Autodesk Inventor part; units mm, degrees
ref_plane "YZ Plane" through (0, 0, 0) normal (1, 0, 0) x (0, 1, 0)
ref_plane "XZ Plane" through (0, 0, 0) normal (0, 1, 0) x (-1, 0, 0)
ref_plane "XY Plane" through (0, 0, 0) normal (0, 0, 1) x (1, 0, 0)
sketch "Sketch1" plane through (0, 0, 0) normal (0, 1, 0) x (-1, 0, 0)
  line L0 (0, 0) -> (45, 0)
  line L1 (45, 0) -> (45, -84)
  line L2 (45, -84) -> (0, -84)
  line L3 (0, -84) -> (0, 0)
  line L4 (0, 0) -> (45, 0)
  line L5 (0, 2) -> (0, 0)
  circle A0 centre (6, -74) radius 2
  circle A1 centre (39, -74) radius 2
  line L6 (22.5, 0) -> (22.5, -84)
  line L7 (45, -10) -> (0, -10)
  line L8 (6, -3.5) -> (10.7625, -3.5)
  line L9 (10.7625, -3.5) -> (10.7625, -5)
  line L10 (10.7625, -5) -> (6, -5)
  line L11 (6, -5) -> (6, -3.5)
  line L12 (6, -16.5) -> (10.7625, -16.5)
  line L13 (10.7625, -16.5) -> (10.7625, -15)
  line L14 (10.7625, -15) -> (6, -15)
  line L15 (6, -15) -> (6, -16.5)
  line L16 (39, -3.5) -> (34.2375, -3.5)
  line L17 (34.2375, -3.5) -> (34.2375, -5)
  line L18 (34.2375, -5) -> (39, -5)
  line L19 (39, -5) -> (39, -3.5)
  line L20 (34.2375, -16.5) -> (34.2375, -15)
  line L21 (39, -15) -> (39, -16.5)
  line L22 (39, -16.5) -> (34.2375, -16.5)
  line L23 (34.2375, -15) -> (39, -15)
  dimension "d0" = 45
  dimension "d1" = 84
  dimension "d3" = 10
  dimension "d4" = 6
  dimension "d5" = 10
  dimension "d6" = 6
  dimension "d7" = 4
  dimension "d8" = 4
  dimension "d19" = 20
  dimension "d20" = 6
  dimension "d21" = 10
  dimension "d22" = 1.5
extrude "Extrusion4" add sketch "Sketch1" along normal blind 1
properties part number "Platte1_2"
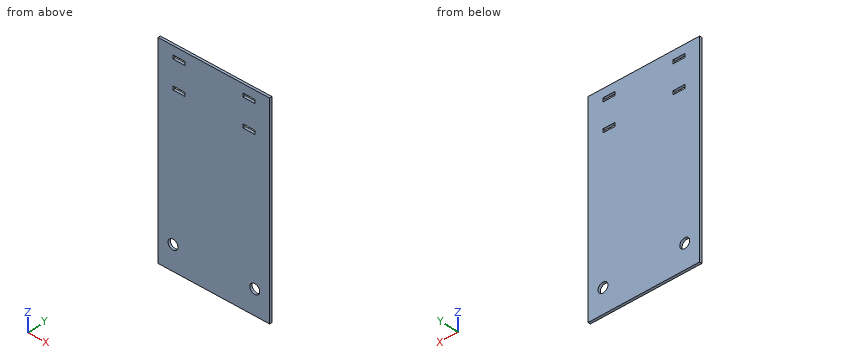
Part model, mm, in its own coordinate system. Coordinates: 2 decimals unless noted, no trailing zeros. Order: outer loops, then holes, each group sorted by start corner. A loop starts at its lowest first (then second) coordinate and runs counter-clockwise, first axis right, second up. Notation, with made-up numbers: (-12.5, 45.5) - (8.5, 45.5) arc R20 cw to (8.5, 72.5) - close; hole circle Ø7 at (44, 62). An arc over 180 degrees is marked (long way). Return JSON: item names as keys, results as strings. Group by question number.
Item 1: Drill centre lines: probe 1 along X at (y, z) = (0.05, -73.5); probe 2 along Z at (x, y) = (-39.5, 0.2). Where is each one in solid material? Low to high. Write a range as from..to.
Item 2: Cut at A-A (z = -74). List the corners of the cut face in (x, y).
Item 3: Pin check, flat tips, straight feed: pin 1 (2.5 mm diameter, centred on x = -39, z = -74, fed in from -Y); pin 2 (1 mm diameter, centred on x = -11, z = -51.5, fed in from -Y). Stop position of each tip, or through.
Check values:
{
 "1": {"probe 1": "x = -45..-40.94, -37.06..-7.94, -4.06..0", "probe 2": "z = -84..-75.94, -72.06..0"},
 "2": {"outline": "(-45, 0) - (-41, 0) - (-41, 1) - (-45, 1) - close; (-37, 0) - (-8, 0) - (-8, 1) - (-37, 1) - close; (-4, 0) - (0, 0) - (0, 1) - (-4, 1) - close"},
 "3": {"pin 1": "passes through", "pin 2": "stops at y = 0"}
}
